Work out the finished part from the listing and answer in its coordinate system (mm). A direction names the side the tool comes from. Coordinates: 2 decimals unless noted, no trailing zeros. Write each loop counter-clockwise with the first axis right and the second up, starting at its lowest first coordinate (ties: lowest second). Pieces come first, ordered by that corner, then holes. Notation, with made-up numbers: (17, -29.75) - (22, -29.75) arc R21 cw to (22, 6.25) - close; hole circle Ø9 at (-22.5, 70.25). An arc over 180 degrees is marked (long way). Use a Markdown table: item, result. Add a question column.
(1) The part is cut by section B-B, the plane y = 575. Give the vertices of the cut face in (x, z).
(2) The part is cut by section D-D, the plane y = 531. Give the vertices of the cut face in (x, z), then the cut area to 3 significant figures.
(3) A tool of negligible diameter and unlimited length cuts with its end or side. For faces 3 (the face through (-99.78, 559.75, 0.76)), 4 (the face through (-55, 560, 0)), from which of +Z, -Z, +X, -X, +Y, -Y can it reach the whole face along a straight path? Write none if from no direction.
(4) The part is cut by section A-A, the plane x = 4.5. Give the vertices of the cut face in (y, z).
(5) For a pull along X with two mould halves and no side action, classify faces 1 (the face through (-46.347, 577.015, 0.76)), 2 (the face through (-55, 560, 1.5)) as released by +X, released by -X, zero draft, split by the parting line, or undercut.
(6) The part is cut by section C-C, the plane x = -41.5. Give the vertices of the cut face in (y, z), then the cut area to 3 significant figures.
(7) Find the intervals of material crossed by line 1 (Y direction, x = 4.5, z = 0.8); line 2 (Y direction, x = -9.5, z = 0.8); line 3 (Y direction, x = -37.5, z = 1.4), in increasing order. Write a range as from..to.
from build123d import *

# Parameters (mm, degrees)
BOSS_EXTRUDE1_DEPTH = 1.5
SKETCH2_R           = 1.6
CUT_EXTRUDE1_DEPTH  = 3.5
CUT_EXTRUDE3_DEPTH  = 10


with BuildPart() as part:
    # Sketch1 → Boss-Extrude1 (new body)
    with BuildSketch(Plane.XY):
        Polygon((-117.914742868, 608.080871166), (-117.914742868, 536.530029297), (-92.914742868, 511.530029297), (10.5, 511.530029297), (10.5, 608.080871166), align=None)
        Polygon((-4.5, 523.530029297), (-4.5, 546.530029297), (-102.914742868, 546.530029297), (-102.914742868, 538.500592045), (-87.94418012, 523.530029297), align=None, mode=Mode.SUBTRACT)
    extrude(amount=BOSS_EXTRUDE1_DEPTH)

    # Sketch2 → Cut-Extrude1 (cut)
    with BuildSketch(Plane.XY.offset(1.5)):
        with Locations((-111.914742868, 539.015310671)):
            Circle(SKETCH2_R)
        with Locations((-90.429461494, 517.530029297)):
            Circle(SKETCH2_R)
        with Locations((-111.914742868, 602.080871166)):
            Circle(SKETCH2_R)
        with Locations((4.5, 602.080871166)):
            Circle(SKETCH2_R)
        with Locations((4.5, 517.530029297)):
            Circle(SKETCH2_R)
    extrude(amount=-CUT_EXTRUDE1_DEPTH, mode=Mode.SUBTRACT)

    # Sketch3 → Cut-Extrude3 (cut)
    with BuildSketch(Plane.XY.offset(1.5)):
        Polygon((-82.4219505, 556.530029297), (-102.914742868, 577.022821666), (-102.914742868, 562.882821666), (-96.5619505, 556.530029297), align=None)
        Polygon((-95.692792369, 598.080871166), (-102.914742868, 598.080871166), (-102.914742868, 591.162821666), (-68.2819505, 556.530029297), (-54.1419505, 556.530029297), align=None)
        Polygon((-67.412792369, 598.080871166), (-81.552792369, 598.080871166), (-40.0019505, 556.530029297), (-25.8619505, 556.530029297), align=None)
        Polygon((-39.132792369, 598.080871166), (-53.272792369, 598.080871166), (-11.7219505, 556.530029297), (-4.5, 556.530029297), (-4.5, 563.448078797), align=None)
        Polygon((-10.852792369, 598.080871166), (-24.992792369, 598.080871166), (-4.5, 577.588078797), (-4.5, 591.728078797), align=None)
    extrude(amount=-CUT_EXTRUDE3_DEPTH, mode=Mode.SUBTRACT)


solid = part.part
Model answer:
| question | item | result |
|---|---|---|
| 1 | outline | (-117.91, 0) - (-102.91, 0) - (-102.91, 1.5) - (-117.91, 1.5) - close; (-100.89, 0) - (-86.75, 0) - (-86.75, 1.5) - (-100.89, 1.5) - close; (-72.61, 0) - (-58.47, 0) - (-58.47, 1.5) - (-72.61, 1.5) - close; (-44.33, 0) - (-30.19, 0) - (-30.19, 1.5) - (-44.33, 1.5) - close; (-16.05, 0) - (10.5, 0) - (10.5, 1.5) - (-16.05, 1.5) - close |
| 2 | outline | (-112.38, 0) - (-95.41, 0) - (-95.41, 1.5) - (-112.38, 1.5) - close; (-4.5, 0) - (10.5, 0) - (10.5, 1.5) - (-4.5, 1.5) - close |
| 2 | area | 48.0 mm^2 |
| 3 | face 3 | +Z, -Z |
| 3 | face 4 | -Z, +X, -X, +Y, -Y |
| 4 | outline | (511.53, 0) - (515.93, 0) - (515.93, 1.5) - (511.53, 1.5) - close; (519.13, 0) - (600.48, 0) - (600.48, 1.5) - (519.13, 1.5) - close; (603.68, 0) - (608.08, 0) - (608.08, 1.5) - (603.68, 1.5) - close |
| 5 | face 1 | undercut |
| 5 | face 2 | zero draft |
| 6 | outline | (511.53, 0) - (523.53, 0) - (523.53, 1.5) - (511.53, 1.5) - close; (546.53, 0) - (558.03, 0) - (558.03, 1.5) - (546.53, 1.5) - close; (572.17, 0) - (586.31, 0) - (586.31, 1.5) - (572.17, 1.5) - close; (598.08, 0) - (608.08, 0) - (608.08, 1.5) - (598.08, 1.5) - close |
| 6 | area | 71.5 mm^2 |
| 7 | line 1 | 511.53..515.93, 519.13..600.48, 603.68..608.08 |
| 7 | line 2 | 511.53..523.53, 546.53..556.53, 568.45..582.59, 596.73..608.08 |
| 7 | line 3 | 511.53..523.53, 546.53..556.53, 568.17..582.31, 596.45..608.08 |
